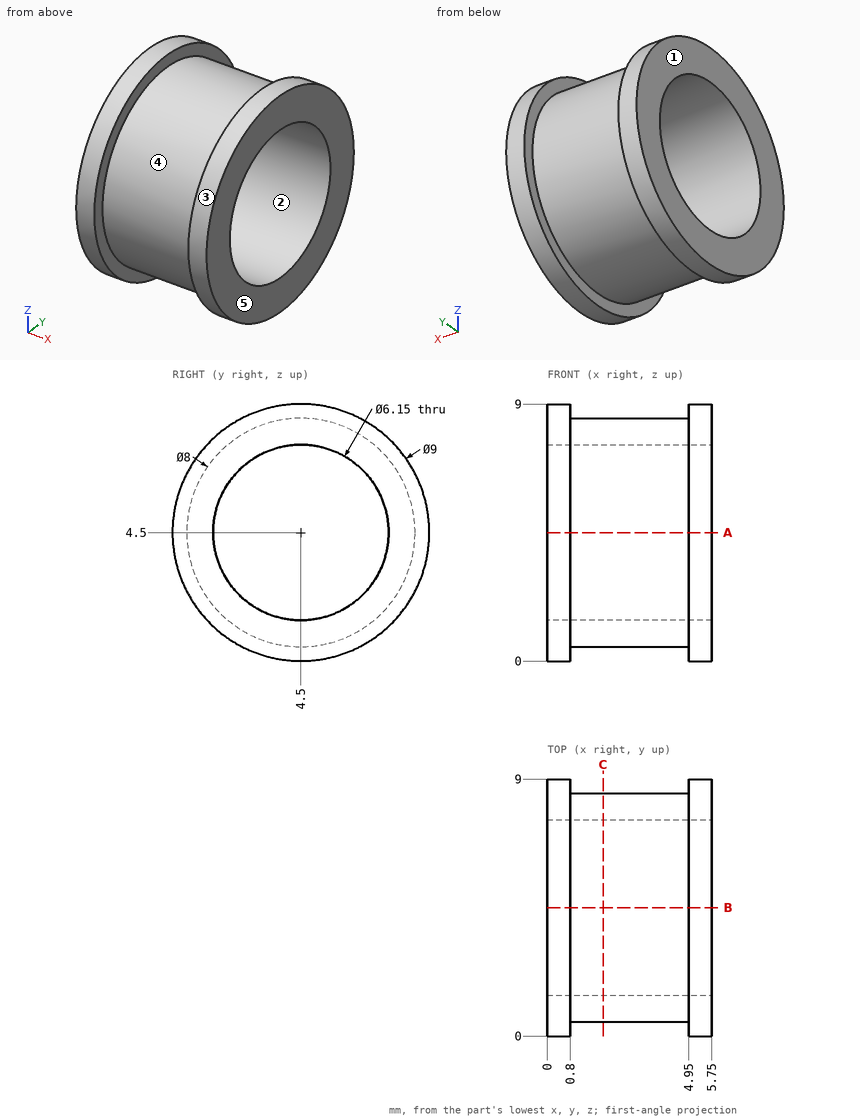
Geometry: see drawing. Coordinates: mm, zero at the bounding-box minimum. A direction names the side the tool comes from. Give positions to 0.01 mm unless a question says otherwise; leave off trailing zeros. Order: outer loops, then holes, each group sorted by start corner. A loop starts at its lowest first (then second) coordinate and runs counter-clockwise, first axis right, second up.
Q1. Ray query, probe 1 along Z at (x, y) = (4.25, 4.5) (3 decimals); probe 2 along X at (y, z) = (7.5, 1.5); probe 3 along Y at (x, z) = (4.8, 1.75). Return the intervals inside material, ascending.
Checked values:
probe 1: z = 0.5 to 1.425, 7.575 to 8.5
probe 2: x = 0 to 0.8, 4.95 to 5.75
probe 3: y = 1.6 to 3.12, 5.88 to 7.4
Q2. Set-up query: the marked faces 4 and 5. Return all of +Z, -Z, +X, -X, +Y, -Y with unobstructed straight access to the full face (end or side cutting, diameter ignored); none if empty.
Checked values:
face 4: none
face 5: +Z, -Z, +X, +Y, -Y
Q3. Section C-C on x = 1.95. Output: boundary loops of the cut face in (y, z) (3 decimals), and give its area (3 significant figures).
Checked values:
outline: circle Ø8 at (4.5, 4.5); hole circle Ø6.15 at (4.5, 4.5)
area: 20.6 mm2
Q4. Section A-A on z = 4.5. Output: boundary loops of the cut face in (x, y) (3 decimals), and give its area (3 significant figures).
Checked values:
outline: (0, 0) - (0.8, 0) - (0.8, 0.5) - (4.95, 0.5) - (4.95, 0) - (5.75, 0) - (5.75, 1.425) - (0, 1.425) - close; (0, 7.575) - (5.75, 7.575) - (5.75, 9) - (4.95, 9) - (4.95, 8.5) - (0.8, 8.5) - (0.8, 9) - (0, 9) - close
area: 12.2 mm2
Q5. Draft query along Y for the marked faces 1, 2 and 3. Return one class per face: +Y half, -Y half, draft (parallel to the pull), parting line (faces both ways), or undercut.
Checked values:
face 1: draft
face 2: undercut
face 3: parting line
Q6. Contact query for flat-ended pins moving along their axis: pin 1 Ø1.5 at (x, z) = (1, 3) entering from -Y; pin 2 Ø5 at (y, z) = (4.5, 4.5) entering from -X; pin 3 Ø4.5 at (y, z) = (6, 5) entering from +X; pin 4 Ø1.5 at (x, z) = (4.5, 3) entering from +Y. Output: stop coordinate, or through.
Checked values:
pin 1: stops at y = 0.07
pin 2: passes through
pin 3: stops at x = 5.75
pin 4: stops at y = 8.91
